Part print with two shaded views. Sizes in mm from the minimum x, y, z corner. A direction names the side the tool comes from. Round coordinates to 2 decimals unless told otherwise and drop trailing zeros. Loops run counter-clockwise (first coordinate to the right, second up) from the corner with the lowest first, then second, coordinate; pieces in that order, holes last. Notation, with made-up numbers: (84, 63.5) - (112, 63.5) arc R22 ccw to (112, 78.5) - close; hole circle Ø5 at (13, -15). An arc over 180 degrees is marked (long way). Use a Markdown table: item, result.
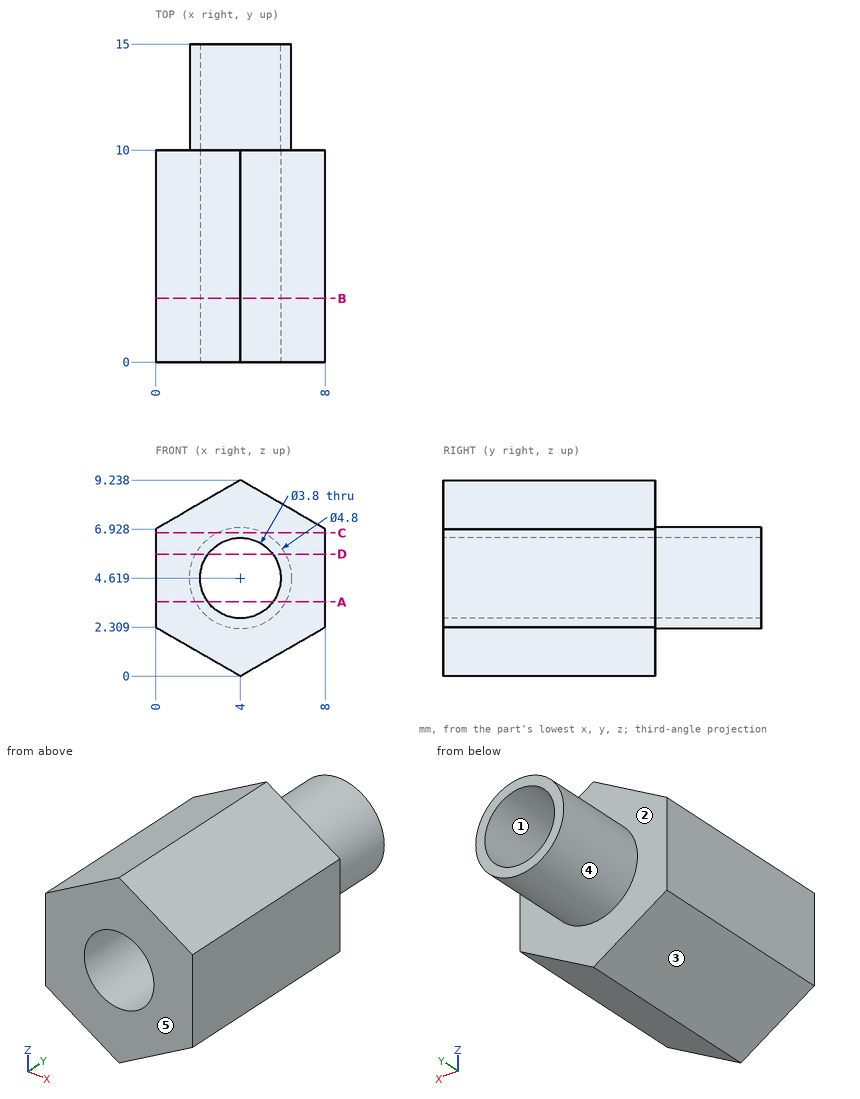
Q1. Cut at B-B, the plane y = 3. List the corners of the cut face in (x, z).
Results found:
| item | result |
|---|---|
| outline | (0, 2.31) - (4, 0) - (8, 2.31) - (8, 6.93) - (4, 9.24) - (0, 6.93) - close; hole circle Ø3.8 at (4, 4.62) |
Q2. Which spindle directions (+Z, -Z, +X, -X, +Y, -Y) get a long thin tool onto all of the face, cutting with end or side? Do the marked faces 4 and 5. Say none if no direction does.
Results found:
| item | result |
|---|---|
| face 4 | +Y |
| face 5 | +Z, -Z, +X, -X, -Y |
Q3. Pull direction X, two halves, no side cores. Call the marked faces 1, 2 and 3: pulls with the +X half, pulls with the -X half, needs draft (parallel to the pull), parting line crosses it, or undercut.
Results found:
| item | result |
|---|---|
| face 1 | undercut |
| face 2 | needs draft |
| face 3 | pulls with the -X half |
Q4. Drop flat-ended pins along their axis: pin 1 (1 mm diameter, centred on x = 1.5, z = 7.5, fed in from -Y); pin 2 (2 mm diameter, centred on x = 6, z = 1.5, fed in from +Y). Give the stop position or say it passes through.
Results found:
| item | result |
|---|---|
| pin 1 | stops at y = 0 |
| pin 2 | stops at y = 10 |
Q5. Probe line 1 (Z direction, x = 4, y = 11.5); line 2 (Y direction, x = 1.75, z = 7.25); line 3 (X direction, y = 5.5, z = 4.5). List the from-to ranges inside material, lowest first.
Results found:
| item | result |
|---|---|
| line 1 | z = 2.22 to 2.72, 6.52 to 7.02 |
| line 2 | y = 0 to 10 |
| line 3 | x = 0 to 2.1, 5.9 to 8 |
Q6. Cut at C-C, the plane z = 6.75. List the corners of the cut face in (x, y).
Results found:
| item | result |
|---|---|
| outline | (0, 0) - (8, 0) - (8, 10) - (5.1, 10) - (5.1, 15) - (2.9, 15) - (2.9, 10) - (0, 10) - close |
Q7. Cut at A-A, the plane z = 3.5. List the corners of the cut face in (x, y) (1 decimal).
Results found:
| item | result |
|---|---|
| outline | (0, 0) - (2.5, 0) - (2.5, 15) - (1.9, 15) - (1.9, 10) - (0, 10) - close; (5.5, 0) - (8, 0) - (8, 10) - (6.1, 10) - (6.1, 15) - (5.5, 15) - close |
Q8. Cut at D-D, the plane z = 5.75. List the corners of the cut face in (x, y).
Results found:
| item | result |
|---|---|
| outline | (0, 0) - (2.47, 0) - (2.47, 15) - (1.88, 15) - (1.88, 10) - (0, 10) - close; (5.53, 0) - (8, 0) - (8, 10) - (6.12, 10) - (6.12, 15) - (5.53, 15) - close |
